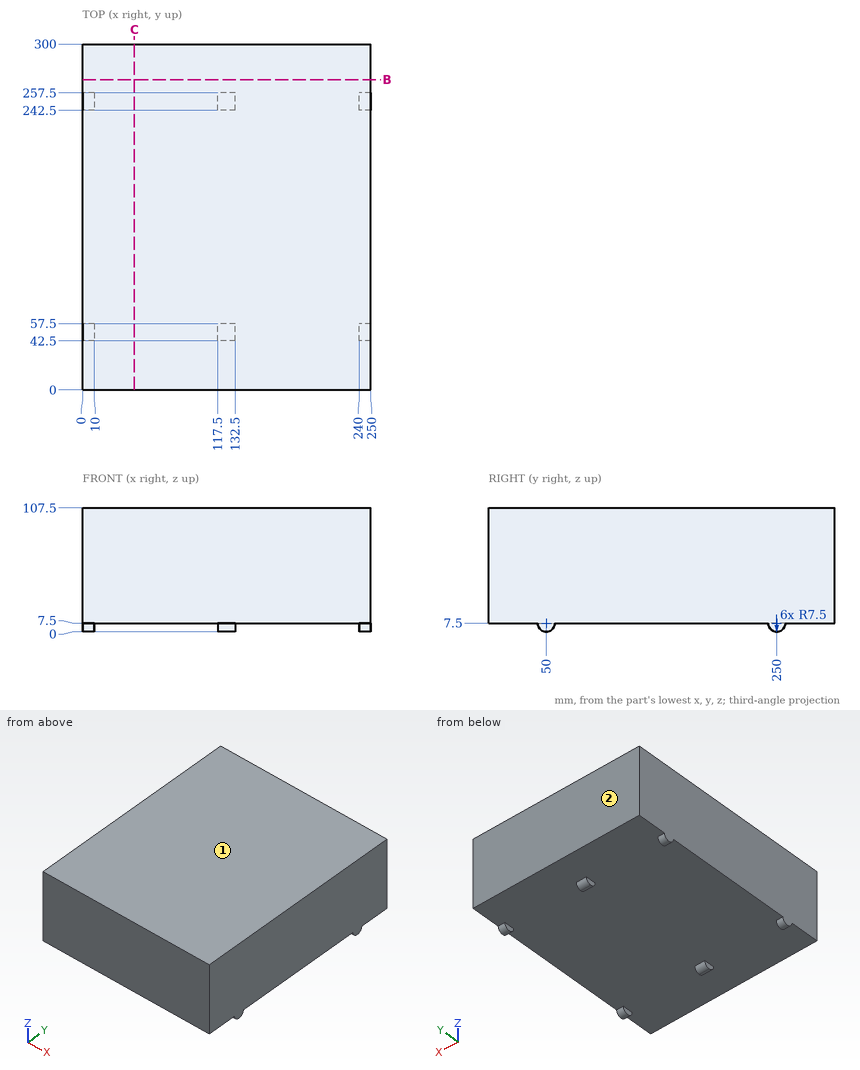
Here's the drawing with two shaded views (mm, measured from the low corner). I have some questions. Coordinates: 2 decimals unless noted, no trailing zeros. Write each loop counter-clockwise with the first axis right and the second up, starting at its lowest first coordinate (ties: lowest second). Pieces come first, ordered by that corner, then holes. Notation, with made-up numbers: (34, 40) - (69, 40) arc R36 ccw to (69, 76) - close; hole circle Ø9 at (84.25, 11). An arc over 180 degrees is marked (long way). Return JSON: item names as keys, results as strings.
Q1. Please list where these lines run through material, in increasing order: L1, parallel to Z at x = 240.5, y = 144.5; L2, parallel to Y at x = 120.5, z = 4; L3, parallel to Z at x = 122.5, y = 245.5. Write a range as from..to.
Computed values:
{"L1": "z = 7.5..107.5", "L2": "y = 43.37..56.63, 243.37..256.63", "L3": "z = 1.5..107.5"}
Q2. I'm going to push a flat-ended pin straight in: pin 1 Ø4 at (x, y) = (129, 263.5) entering from -Z. Where does the tip first touch, or does it pass through?
Computed values:
{"pin 1": "stops at z = 7.5"}
Q3. If we section it at B-B (y = 269): Please give me the cut outline in (x, z).
Computed values:
{"outline": "(0, 7.5) - (250, 7.5) - (250, 107.5) - (0, 107.5) - close"}
Q4. Thinking about a two-plate mould opening in Z: for the marked faces 1 and 2, which applies, +Z half, -Z half, draft (parallel to the pull), parting line (faces both ways), or undercut?
Computed values:
{"face 1": "+Z half", "face 2": "draft"}
Q5. If we section it at C-C (x = 45): Please give me the cut outline in (y, z).
Computed values:
{"outline": "(0, 7.5) - (300, 7.5) - (300, 107.5) - (0, 107.5) - close"}
